from build123d import *

# Parameters (mm, degrees)
SKETCH1_R           = 32
BOSS_EXTRUDE1_DEPTH = 100
SKETCH2_R           = 27
CUT_EXTRUDE1_DEPTH  = 85
SKETCH3_W           = 28
SKETCH3_H           = 28
CUT_EXTRUDE2_DEPTH  = 25


with BuildPart() as part:
    # Sketch1 → Boss-Extrude1 (new body)
    with BuildSketch(Plane(origin=(0, 0, 0), x_dir=(1, 0, 0), z_dir=(0, 1, 0))):
        with Locations(Location((0, 0, 0), (0, 0, 270))):
            Circle(SKETCH1_R)
    extrude(amount=BOSS_EXTRUDE1_DEPTH)

    # Sketch2 → Cut-Extrude1 (cut)
    with BuildSketch(Plane(origin=(0, 100, 0), x_dir=(1, 0, 0), z_dir=(0, 1, 0))):
        with Locations(Location((0, 0, 0), (0, 0, 270))):
            Circle(SKETCH2_R)
    extrude(amount=-CUT_EXTRUDE1_DEPTH, mode=Mode.SUBTRACT)

    # Sketch3 → Cut-Extrude2 (cut)
    with BuildSketch(Plane.XZ):
        Rectangle(SKETCH3_W, SKETCH3_H)
    extrude(amount=-CUT_EXTRUDE2_DEPTH, mode=Mode.SUBTRACT)


solid = part.part
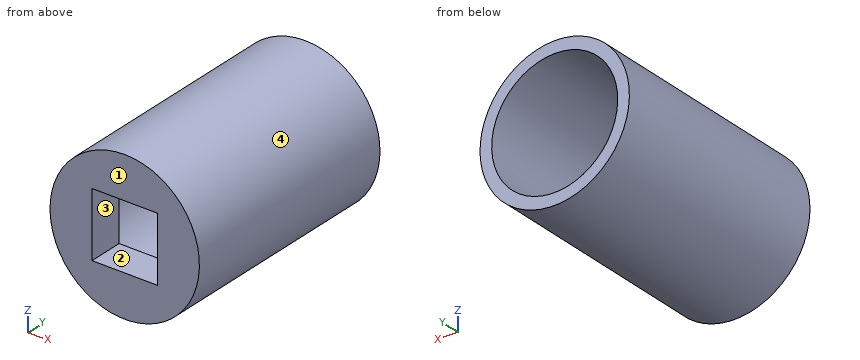
Build history of the part. All positions in model axes, mm. Face numbers are marked on the shaded views. Coordinates: 2 decimals unless noted, no trailing zeros. Write each loop counter-clockwise with the first axis right and the second up, starting at its lowest first coordinate (ties: lowest second). Pieces come first, ordered by that corner, then holes.
(1) Mould opens along Z. For the marked faces 1, 2, 3 and 4 say: pulls with the +Z half, pulls with the -Z half, needs draft (parallel to the pull), parting line crosses it, or undercut.
(2) Cut at D-D on y = 62.5. List the corners of the cut face in (x, z), and give its area (3 significant figures).
(3) Drill centre lines: line 1 (X direction, y = 74, z = 0); line 2 (Z direction, x = -19, y = 56); line 3 (Y direction, x = 10.5, z = -14.5). Where is each one in solid material? Low to high.
(4) Cut at C-C on z = -25. List the corners of the cut face in (x, y), and give its area (3 significant figures).
(5) Cut at A-A on z = 0. List the corners of the cut face in (x, y), and give its area (3 significant figures).
(6) Pin check, flat tips, straight feed: pin 1 Ø2 at (y, z) = (70.5, 14.5) entering from +X; pin 2 Ø1 at (y, z) = (43, 20.5) entering from -X; pin 3 Ø2 at (x, y) = (2, 69.5) entering from -Z. Stop position of each tip, or through.
(7) Cut at B-B on x = 0. List the corners of the cut face in (y, z), and give its area (3 significant figures).
Working result:
1. face 1: needs draft
1. face 2: undercut
1. face 3: undercut
1. face 4: parting line crosses it
2. outline: circle Ø64 at (0, 0); hole circle Ø54 at (0, 0)
2. area: 927 mm2
3. line 1: x = -32 to -27, 27 to 32
3. line 2: z = -25.75 to -19.18, 19.18 to 25.75
3. line 3: y = 0 to 15
4. outline: (-19.97, 0) - (19.97, 0) - (19.97, 100) - (10.2, 100) - (10.2, 15) - (-10.2, 15) - (-10.2, 100) - (-19.97, 100) - close
4. area: 2,260 mm2
5. outline: (-32, 0) - (-14, 0) - (-14, 15) - (-27, 15) - (-27, 100) - (-32, 100) - close; (14, 0) - (32, 0) - (32, 100) - (27, 100) - (27, 15) - (14, 15) - close
5. area: 1,390 mm2
6. pin 1: stops at x = 29.01
6. pin 2: stops at x = -24.98
6. pin 3: stops at z = -31.98
7. outline: (0, -32) - (100, -32) - (100, -27) - (15, -27) - (15, -14) - (0, -14) - close; (0, 14) - (15, 14) - (15, 27) - (100, 27) - (100, 32) - (0, 32) - close
7. area: 1,390 mm2
